Design review of the part built by this model. Coordinates are the model's own, in mm. Face numbers are marked on the shaded views. A direction names the side the tool comes from. Give positions to 0.01 mm unless a question says otherwise; leave off trailing zeros. Loops run counter-clockwise (first coordinate to the right, second up) from the corner with the lowest first, then second, coordinate; pieces in that order, holes last. Notation, with made-up numbers: (38.5, 64.5) -> (79.5, 64.5) arc R22 ccw to (79.5, 87.5) -> close; hole circle Ø1 at (67, 2.5). An arc over 180 degrees is marked (long way). Use CSV: the item, a comma, the result in double quotes. Start each with the question number.
Item 1: Clearance check with flat-ended pins moving along their axes: pin 1 (3 mm diameter, centred on y = 46.5, z = 4, fed in from -X); pin 2 (1 mm diameter, centred on x = 14.5, z = 2, fed in from +Y). State where each tip first meets the part, or that it passes through.
Item 2: We need section A-A (z = 5.5). State the section outline as (x, y) points.
Item 3: We need section C-C (x = 54.5). State the section outline as (y, z) points, plus the area to 3 significant figures.
Item 4: Wall thickness on line 1 along Y through (x, z) = (36, 2); line 2 along Y through (x, z) = (19, 1): over which ranges is each line inside the solid? List them lowest first. Write a range as from..to.
Item 5: We need section D-D (y = 32.5). State the section outline as (x, z) points, plus the area to 3 significant figures.
Item 6: The part is to be moulded in two halves that separate along Y. For the marked faces 4, 5 and 6, say which applies: +Y half, -Y half, draft (parallel to the pull), parting line (faces both ways), or undercut.
Item 7: We need section B-B (x = 36). State the section outline as (y, z) points, plus the area to 3 significant figures.
Item 8: For the marked faces 1, 2 and 3, list the 3-axis set-ups (+Z, -Z, +X, -X, +Y, -Y) from which the entire face can be reached by the end or side of a thin tool; tool diameter is ignored.
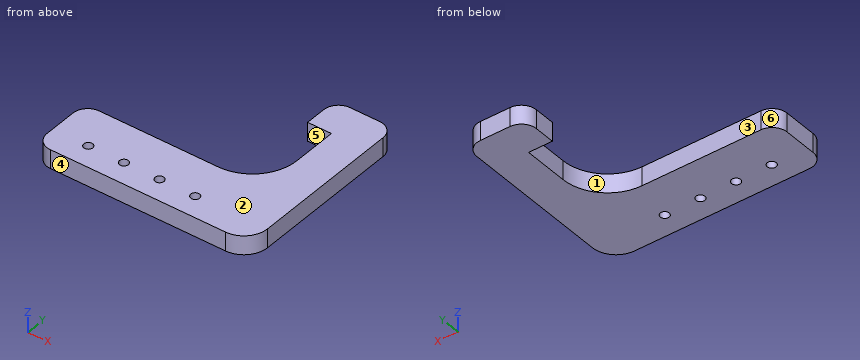
from build123d import *

# Parameters (mm, degrees)
SKETCH1_W           = 60
SKETCH1_H           = 21.35
SKETCH1_R           = 1.5
BOSS_EXTRUDE1_DEPTH = 6.35
FILLET1_R           = 15
FILLET3_R           = 5
FILLET5_R           = 5
FILLET6_R           = 5
FILLET7_R           = 8


with BuildPart() as part:
    # Sketch1 → Boss-Extrude1 (new body)
    with BuildSketch(Plane.XY):
        with Locations((30, 10.675)):
            Rectangle(SKETCH1_W, SKETCH1_H)
        with Locations((12, 7.5)):
            Circle(SKETCH1_R, mode=Mode.SUBTRACT)
        with Locations((24, 7.5)):
            Circle(SKETCH1_R, mode=Mode.SUBTRACT)
        with Locations((36, 7.5)):
            Circle(SKETCH1_R, mode=Mode.SUBTRACT)
        with Locations((48, 7.5)):
            Circle(SKETCH1_R, mode=Mode.SUBTRACT)
        Polygon((60, 21.35), (60, 0), (72, 0), (72, 51.35), (60, 51.35), align=None)
        Polygon((52, 51.35), (60, 51.35), (72, 51.35), (72, 63.35), (52, 63.35), align=None)
    extrude(amount=BOSS_EXTRUDE1_DEPTH)

    # Fillet1
    fillet1_edges = [part.edges().sort_by_distance(p)[0] for p in [
        (60, 21.35, 3.175),
    ]]
    fillet(fillet1_edges, radius=FILLET1_R)

    # Fillet3
    fillet3_edges = [part.edges().sort_by_distance(p)[0] for p in [
        (52, 63.35, 3.175),
    ]]
    fillet(fillet3_edges, radius=FILLET3_R)

    # Fillet5
    fillet5_edges = [part.edges().sort_by_distance(p)[0] for p in [
        (0, 0, 3.175),
        (0, 21.35, 3.175),
    ]]
    fillet(fillet5_edges, radius=FILLET5_R)

    # Fillet6
    fillet6_edges = [part.edges().sort_by_distance(p)[0] for p in [
        (72, 63.35, 3.175),
    ]]
    fillet(fillet6_edges, radius=FILLET6_R)

    # Fillet7
    fillet7_edges = [part.edges().sort_by_distance(p)[0] for p in [
        (72, 0, 3.175),
    ]]
    fillet(fillet7_edges, radius=FILLET7_R)


solid = part.part
Results found:
1,pin 1,"x = 60"
1,pin 2,"y = 21.35"
2,outline,"(0, 5) arc R5 ccw to (5, 0) -> (64, 0) arc R8 ccw to (72, 8) -> (72, 58.35) arc R5 ccw to (67, 63.35) -> (57, 63.35) arc R5 ccw to (52, 58.35) -> (52, 51.35) -> (60, 51.35) -> (60, 36.35) arc R15 cw to (45, 21.35) -> (5, 21.35) arc R5 ccw to (0, 16.35) -> close; hole circle Ø3 at (12, 7.5); hole circle Ø3 at (24, 7.5); hole circle Ø3 at (36, 7.5); hole circle Ø3 at (48, 7.5)"
3,outline,"(0, 0) -> (24.74, 0) -> (24.74, 6.35) -> (0, 6.35) -> close; (51.35, 0) -> (62.68, 0) -> (62.68, 6.35) -> (51.35, 6.35) -> close"
3,area,"229 mm²"
4,line 1,"0..6, 9..21.35"
4,line 2,"0..21.35"
5,outline,"(59.5, 0) -> (72, 0) -> (72, 6.35) -> (59.5, 6.35) -> close"
5,area,"79.4 mm²"
6,face 4,"-Y half"
6,face 5,"undercut"
6,face 6,"+Y half"
7,outline,"(0, 0) -> (6, 0) -> (6, 6.35) -> (0, 6.35) -> close; (9, 0) -> (21.35, 0) -> (21.35, 6.35) -> (9, 6.35) -> close"
7,area,"117 mm²"
8,face 1,"+Z, -Z, -X"
8,face 2,"+Z, +X, -X, +Y, -Y"
8,face 3,"+Z, -Z, -X, +Y"
